Check sheet for the modelled part. Datum: model origin and axes. Units: mm. Face numbers are marked on the shaded views. A direction names the side the tool comes from. Round coordinates to 2 decimals unless told otherwise and drop trailing zeros. Loops run counter-clockwise (first coordinate to the right, second up) from the corner with the lowest first, then second, coordinate; pieces in that order, holes last. Notation, with made-up numbers: (11, 10.5) -> (17, 10.5) arc R13 cw to (17, 32.5) -> close; hole circle Ø2 at (-29.5, 13). An arc over 180 degrees is marked (long way). One line per item, written item: value. Start each with the question number.
1. Go/stop test with flat-tipped pins: pin 1 (2 mm diameter, centred on x = -52.5, z = -9, fed in from +Y); pin 2 (4 mm diameter, centred on y = -15.5, z = -4.5, fed in from -X); pin 3 (7.5 mm diameter, centred on x = 73.025, y = 0, fed in from +Z); pin 4 (2 mm diameter, centred on y = 42, z = -0.5, fed in from +X). Record where each tip stops, or that it passes through.
2. Cross-section at C-C on z = 1.5. Record the cut outline in (x, y) (1 decimal), then the cut area to 3 significant figures.
3. Set-up check for the marked faces 4, 5 and 6: record each of +Z, -Z, +X, -X, +Y, -Y from which the full face is reachable in a straight line by a thin tool's end or side.
4. Release check for a two-part mould opening along Z. For the marked faces 1, 2 and 3 record: +Z half, -Z half, draft (parallel to the pull), parting line (faces both ways), or undercut.
5. Material ranges on L1, parallel to Y at x = 0, z = -0.5 (3 decimals); L2, parallel to Z at x = -9.5, y = 70 (3 decimals); L3, parallel to X at y = 20.5, z = -2.5, recorded low to high.
6. Cross-section at D-D on y = 67. Record the cut outline in (x, z) (3 decimals), then the cut area to 3 significant figures.
7. Cross-section at B-B on x = 0. Record the cut outline in (y, z) (3 decimals).
8. Cross-section at A-A on y = 0. Count the separate pieces of the cut face and the enclosed holes in it, then the cut area to 3 significant figures.
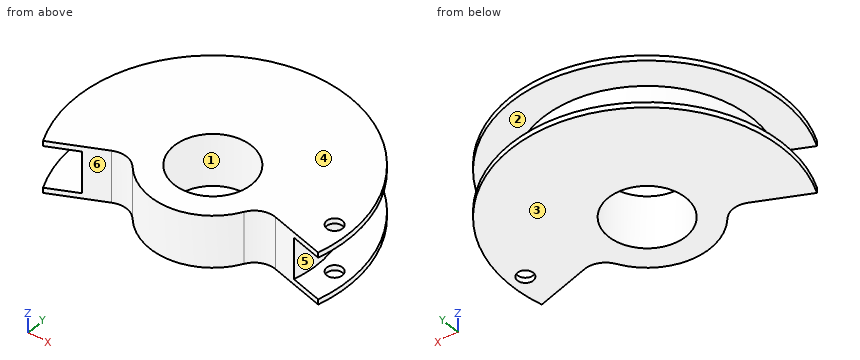
from build123d import *

# Parameters (mm, degrees)
F2_R     = 4.7625
F3_DEPTH = 50.8
F5_DEPTH = 31.751
F6_R     = 12.7


with BuildPart() as f1:
    # F0 (on Front) → F1 (revolve)
    with BuildSketch(Plane.XZ):
        Polygon((29.845, 15.875), (23.495, 15.875), (23.495, -15.875), (29.845, -15.875), (60.325, -15.875), (82.55, -15.875), (82.55, -12.7), (63.5, -12.7), (63.5, 12.7), (82.55, 12.7), (82.55, 15.875), (60.325, 15.875), align=None)
    revolve(axis=Axis((0, 0, 17.235907), (0, 0, 1)))

    # F2 (on Top) → F3 (cut, symmetric)
    with BuildSketch(Plane.XY):
        with Locations((73.025, 0)):
            Circle(F2_R)
    extrude(amount=F3_DEPTH, both=True, mode=Mode.SUBTRACT)

    # F4 (on face) → F5 (cut, through all)
    with BuildSketch(Plane.XY.offset(15.875)):
        with BuildLine():
            ThreePointArc((-74.815708, -34.887138), (7.194707, -82.235872), (79.737177, -21.365512))
            Line((79.737177, -21.365512), (36.801774, -9.861006))
            ThreePointArc((36.801774, -9.861006), (3.320634, -37.955018), (-34.530327, -16.101756))
            Line((-34.530327, -16.101756), (-74.815708, -34.887138))
        make_face()
    extrude(amount=-F5_DEPTH, mode=Mode.SUBTRACT)

    # F6
    f6_edges = [f1.edges().sort_by_distance(p)[0] for p in [
        (-34.530327, -16.101756, 0),
        (36.801774, -9.861006, 0),
    ]]
    fillet(f6_edges, radius=F6_R)


solid = f1.part
Taken from the geometry:
1. pin 1: stops at y = 37.15
1. pin 2: stops at x = -62.05
1. pin 3: passes through
1. pin 4: stops at x = 48.49
2. outline: (-57.6, -26.8) -> (-44.6, -20.8) arc R12.7 cw to (-29.4, -24.2) arc R38.1 ccw to (33.2, -18.7) arc R12.7 cw to (47.5, -12.7) -> (61.3, -16.4) arc R63.5 ccw (long way) to start; hole circle Ø47 at (0, 0)
2. area: 7,830 mm2
3. face 4: +Z, +X, -X, +Y, -Y
3. face 5: none
3. face 6: +Z, -Z, -Y
4. face 1: draft
4. face 2: undercut
4. face 3: -Z half
5. L1: y = -38.1 to -23.495, 23.495 to 63.5
5. L2: z = -15.875 to -12.7, 12.7 to 15.875
5. L3: x = -60.1 to -11.48, 11.48 to 60.1
6. outline: (-48.223, -15.875) -> (48.223, -15.875) -> (48.223, -12.7) -> (-48.223, -12.7) -> close; (-48.223, 12.7) -> (48.223, 12.7) -> (48.223, 15.875) -> (-48.223, 15.875) -> close
6. area: 612 mm2
7. outline: (-38.1, -15.875) -> (-23.495, -15.875) -> (-23.495, 15.875) -> (-38.1, 15.875) -> close; (23.495, -15.875) -> (82.55, -15.875) -> (82.55, -12.7) -> (63.5, -12.7) -> (63.5, 12.7) -> (82.55, 12.7) -> (82.55, 15.875) -> (23.495, 15.875) -> close
8. separate pieces: 4
8. enclosed holes: 0
8. area: 2,720 mm2
